Input: part model. Units: mm. Frame: model coordinates. A direction names the side the tool comes from. Round coordinates to 2 decimals unless told otherwise and drop trailing zeros. Order: outer loops, then holes, each group sorted by start corner. A loop starts at its lowest first (then second) coordinate and runs counter-clockwise, first axis right, second up. Notation, with made-up numbers: (-27, 89) -> (23, 89) arc R21 cw to (23, 99) -> close; hole circle Ø7 at (-31.5, 68). An arc over 180 degrees is marked (long way). Use a Markdown table: item, result.
from build123d import *

# Parameters (mm, degrees)
SKETCH1_W           = 45
SKETCH1_H           = 20
BOSS_EXTRUDE1_DEPTH = 1.5
BOSS_EXTRUDE2_DEPTH = 3
SKETCH4_R           = 8
BOSS_EXTRUDE3_DEPTH = 12
SKETCH5_R           = 6.5
CUT_EXTRUDE1_DEPTH  = 1
SKETCH6_R           = 1
BOSS_EXTRUDE4_DEPTH = 2
FILLET1_R           = 0.5
CUT_EXTRUDE2_REACH  = 29.391
SKETCH3_R           = 0.83
SKETCH7_W           = 9.858526848
SKETCH7_H           = 2.639541059
BOSS_EXTRUDE5_DEPTH = 2.5


with BuildPart() as part:
    # Sketch1 → Boss-Extrude1 (new body)
    with BuildSketch(Plane(origin=(0, 0, 0), x_dir=(1, 0, 0), z_dir=(0, 1, 0))):
        Rectangle(SKETCH1_W, SKETCH1_H)
    extrude(amount=BOSS_EXTRUDE1_DEPTH)

    # Sketch2 → Boss-Extrude2 (add)
    with BuildSketch(Plane(origin=(0, 1.5, 0), x_dir=(1, 0, 0), z_dir=(0, 1, 0))):
        with BuildLine():
            Line((-3, 5.25), (3, 5.25))
            ThreePointArc((3, 5.25), (5, 7.25), (3, 9.25))
            Line((3, 9.25), (-3, 9.25))
            ThreePointArc((-3, 9.25), (-5, 7.25), (-3, 5.25))
        make_face()
    extrude(amount=BOSS_EXTRUDE2_DEPTH)

    # Sketch4 → Boss-Extrude3 (add)
    with BuildSketch(Plane(origin=(0, 1.5, 0), x_dir=(1, 0, 0), z_dir=(0, 1, 0))):
        with Locations(Location((-13, 0, 0), (0, 0, 90))):
            Circle(SKETCH4_R)
        with Locations(Location((13, 0, 0), (0, 0, 90))):
            Circle(SKETCH4_R)
    extrude(amount=BOSS_EXTRUDE3_DEPTH)

    # Sketch5 → Cut-Extrude1 (cut)
    with BuildSketch(Plane(origin=(0, 13.5, 0), x_dir=(1, 0, 0), z_dir=(0, 1, 0))):
        with Locations(Location((-13, 0, 0), (0, 0, 270))):
            Circle(SKETCH5_R)
        with Locations(Location((13, 0, 0), (0, 0, 270))):
            Circle(SKETCH5_R)
    extrude(amount=-CUT_EXTRUDE1_DEPTH, mode=Mode.SUBTRACT)

    # Sketch6 → Boss-Extrude4 (add)
    with BuildSketch(Plane(origin=(0, 1.5, 0), x_dir=(1, 0, 0), z_dir=(0, 1, 0))):
        with Locations(Location((-3.81, -8.6, 0), (0, 0, 90))):
            Circle(SKETCH6_R)
        with Locations(Location((-1.27, -8.6, 0), (0, 0, 90))):
            Circle(SKETCH6_R)
        with Locations(Location((1.27, -8.6, 0), (0, 0, 90))):
            Circle(SKETCH6_R)
        with Locations(Location((3.81, -8.6, 0), (0, 0, 90))):
            Circle(SKETCH6_R)
    extrude(amount=BOSS_EXTRUDE4_DEPTH)

    # Fillet1
    fillet1_edges = [part.edges().sort_by_distance(p)[0] for p in [
        (-13, 13.5, 8),
        (13, 13.5, 8),
    ]]
    fillet(fillet1_edges, radius=FILLET1_R)

    # Sketch3 → Cut-Extrude2 (cut, up to next)
    with BuildSketch(Plane(origin=(0, 1.5, 0), x_dir=(1, 0, 0), z_dir=(0, 1, 0)), mode=Mode.PRIVATE) as cut_extrude2_sk1:
        with Locations(Location((-21, 8.6, 0), (0, 0, 270))):
            Circle(SKETCH3_R)
    cut_extrude2_tool1 = extrude(cut_extrude2_sk1.sketch, amount=-CUT_EXTRUDE2_REACH, mode=Mode.PRIVATE) & part.part
    # Sketch3 → Cut-Extrude2 (cut, up to next)
    with BuildSketch(Plane(origin=(0, 1.5, 0), x_dir=(1, 0, 0), z_dir=(0, 1, 0)), mode=Mode.PRIVATE) as cut_extrude2_sk2:
        with Locations(Location((-21, -8.6, 0), (0, 0, 270))):
            Circle(SKETCH3_R)
    cut_extrude2_tool2 = extrude(cut_extrude2_sk2.sketch, amount=-CUT_EXTRUDE2_REACH, mode=Mode.PRIVATE) & part.part
    # Sketch3 → Cut-Extrude2 (cut, up to next)
    with BuildSketch(Plane(origin=(0, 1.5, 0), x_dir=(1, 0, 0), z_dir=(0, 1, 0)), mode=Mode.PRIVATE) as cut_extrude2_sk3:
        with Locations(Location((21, -8.6, 0), (0, 0, 270))):
            Circle(SKETCH3_R)
    cut_extrude2_tool3 = extrude(cut_extrude2_sk3.sketch, amount=-CUT_EXTRUDE2_REACH, mode=Mode.PRIVATE) & part.part
    # Sketch3 → Cut-Extrude2 (cut, up to next)
    with BuildSketch(Plane(origin=(0, 1.5, 0), x_dir=(1, 0, 0), z_dir=(0, 1, 0)), mode=Mode.PRIVATE) as cut_extrude2_sk4:
        with Locations(Location((21, 8.6, 0), (0, 0, 270))):
            Circle(SKETCH3_R)
    cut_extrude2_tool4 = extrude(cut_extrude2_sk4.sketch, amount=-CUT_EXTRUDE2_REACH, mode=Mode.PRIVATE) & part.part
    add(cut_extrude2_tool1.solids().sort_by_distance((-21, 1.5, -8.6))[0], mode=Mode.SUBTRACT)
    add(cut_extrude2_tool2.solids().sort_by_distance((-21, 1.5, 8.6))[0], mode=Mode.SUBTRACT)
    add(cut_extrude2_tool3.solids().sort_by_distance((21, 1.5, 8.6))[0], mode=Mode.SUBTRACT)
    add(cut_extrude2_tool4.solids().sort_by_distance((21, 1.5, -8.6))[0], mode=Mode.SUBTRACT)

    # Sketch7 → Boss-Extrude5 (add)
    with BuildSketch(Plane.XZ):
        with Locations((0, 8.580229471)):
            Rectangle(SKETCH7_W, SKETCH7_H)
    extrude(amount=BOSS_EXTRUDE5_DEPTH)


solid = part.part
1) Cut plane B-B on x = -13. Return loops of the section in (y, z), and give its area (3 significant figures).
Answer key:
| item | result |
|---|---|
| outline | (0, -10) -> (1.5, -10) -> (1.5, -8) -> (13, -8) arc R0.5 ccw to (13.5, -7.5) -> (13.5, -6.5) -> (12.5, -6.5) -> (12.5, 6.5) -> (13.5, 6.5) -> (13.5, 7.5) arc R0.5 ccw to (13, 8) -> (1.5, 8) -> (1.5, 10) -> (0, 10) -> close |
| area | 209 mm^2 |
2) Draft query along X for faces 1 (the face through (22.5, 1, 0)), 2 (the face through (0, -2.5, 9)), 3 (the face through (-21.74, 0.76, -8.22)). Return one class per face: released by +X, released by -X, zero draft, split by the parting line, or undercut.
Answer key:
| item | result |
|---|---|
| face 1 | released by +X |
| face 2 | zero draft |
| face 3 | undercut |
3) Contact query for flat-ended pins moving along their axis: P1, Ø1.5, axis at x = 1.5, y = 3, coming from the +Z side; P2, Ø3, axis at y = -0.5, z = -3.5, coming from the -X side; P3, Ø4, axis at x = -0.5, y = 5, coming from the -Z side; P4, Ø4, axis at y = 12, z = -3.5, coming from the +X side. Output: stop coordinate, or through.
Answer key:
| item | result |
|---|---|
| P1 | stops at z = 9.6 |
| P2 | stops at x = -22.5 |
| P3 | stops at z = -9.25 |
| P4 | stops at x = 20.86 |
4) Ray query, probe 1 along X at (y, z) = (0.8, 8.6); probe 2 along Y at (x, z) = (12.5, 5.75); probe 3 along Y at (x, z) = (9, -9). Return the intervals inside material, ascending.
Answer key:
| item | result |
|---|---|
| probe 1 | x = -22.5 to -21.83, -20.17 to 20.17, 21.83 to 22.5 |
| probe 2 | y = 0 to 12.5 |
| probe 3 | y = 0 to 1.5 |
5) Cut plane C-C on z = 0. Return loops of the section in (x, y), and give its area (3 significant figures).
Answer key:
| item | result |
|---|---|
| outline | (-22.5, 0) -> (22.5, 0) -> (22.5, 1.5) -> (21, 1.5) -> (21, 13) arc R0.5 ccw to (20.5, 13.5) -> (19.5, 13.5) -> (19.5, 12.5) -> (6.5, 12.5) -> (6.5, 13.5) -> (5.5, 13.5) arc R0.5 ccw to (5, 13) -> (5, 1.5) -> (-5, 1.5) -> (-5, 13) arc R0.5 ccw to (-5.5, 13.5) -> (-6.5, 13.5) -> (-6.5, 12.5) -> (-19.5, 12.5) -> (-19.5, 13.5) -> (-20.5, 13.5) arc R0.5 ccw to (-21, 13) -> (-21, 1.5) -> (-22.5, 1.5) -> close |
| area | 425 mm^2 |
6) Cut plane A-A on z = 8.6. State how many separate pieces and enclosed holes the cut face has, and give its area (3 significant figures).
Answer key:
| item | result |
|---|---|
| separate pieces | 3 |
| enclosed holes | 0 |
| area | 103 mm^2 |
7) Cut plane D-D on y = 7.5. Return loops of the section in (x, z), and give its area (3 significant figures).
Answer key:
| item | result |
|---|---|
| outline | circle Ø16 at (-13, 0); circle Ø16 at (13, 0) |
| area | 402 mm^2 |
8) Set-up query: faces 4 (the face through (-4, 3.5, 9)), 5 (the face through (20.81, 7.17, 1.73)), 6 (the face through (0, 4.5, -7)). Return all of +Z, -Z, +X, -X, +Y, -Y with unobstructed straight access to the full face (end or side cutting, diameter ignored); none if empty.
Answer key:
| item | result |
|---|---|
| face 4 | +Z, +Y |
| face 5 | +Y |
| face 6 | +Z, -Z, +Y |
